For this review, take the finished solid that the model builds, in its own axes (mm). A direction names the side the tool comes from. Give positions to 0.01 mm unless a question says otherwise; leave off trailing zeros. Write each loop counter-clockwise with the first axis right and the second up, starting at its lowest first coordinate (ties: lowest second). Pieces come first, ordered by that corner, then holes. Notation, with made-up numbers: M 47,65 L 66,65 A12 ccw 66,80 Z; hole C 10,71.25 d11. An arc over 180 degrees is marked long. Use one line per item in the form item = value. Start each with the question number.
Q1. Consider section A-A on z = 28. Write out the cut boundary in (x, y).
Q2. Consider section D-D on z = 125. Write out the cut boundary in (x, y).
Q3. Consider section C-C on y = -73. Write out the cut boundary in (x, z).
Q4. For probe 1 along Z at (x, y) = (137.5, -93.5); probe 2 along Y at (x, z) = (129, 45.5), list the stretches that pass through material, from the lowest coordinate up. Write a range as [from, to].
Q5. Tool access review of faces 1 (the flat face through (-101, 1, 50.8)), 2 (the flat face through (-49, -50.8, 101)), 3 (the flat face through (101, -50.8, -1)): name each direction out of +Z, -Z, +X, -X, +Y, -Y from which nothing blocks a thin tool from reaching the whole face with its end or side.
Q6. Consider section B-B on x = 26. Write out the cut boundary in (y, z).
Q7. Clearance check with flat-ended pins moving along their axes: pin 1 Ø1 at (y, z) = (-40.5, -30.5) entering from -X; pin 2 Ø1 at (y, z) = (10.5, 11.5) entering from +X. State where each tip first meets the part, or that it passes through.
```python
from build123d import *

# Parameters (mm, degrees)
F1_W      = 101.6
F1_H      = 101.6
F2_DEPTH  = 50.8
F3_W      = 101.6
F3_H      = 101.6
F4_DEPTH  = 101.6
F5_W      = 101.6
F5_H      = 101.6
F6_DEPTH  = 101.6
F7_W      = 101.6
F7_H      = 101.6
F8_DEPTH  = 101.6
F9_W      = 101.6
F9_H      = 101.6
F10_DEPTH = 101.6


# Not quite as in the source:
# - a variable given as a bare number and used for a length is read in inches; the dataset says mm whatever the document's units were


with BuildPart() as f2:
    # F1 (on Front) → F2 (new body, symmetric)
    with BuildSketch(Plane.XZ):
        Rectangle(F1_W, F1_H)
    extrude(amount=F2_DEPTH, both=True)

    # F3 (on face) → F4 (join)
    with BuildSketch(Plane.XZ.offset(50.8)):
        Rectangle(F3_W, F3_H)
    extrude(amount=F4_DEPTH)

    # F5 (on face) → F6 (join)
    with BuildSketch(Plane.YZ.offset(50.8)):
        with Locations((-101.6, 0)):
            Rectangle(F5_W, F5_H)
    extrude(amount=F6_DEPTH)

    # F7 (on face) → F8 (join)
    with BuildSketch(Plane.XY.offset(50.8)):
        Rectangle(F7_W, F7_H)
    extrude(amount=F8_DEPTH)

    # F9 (on face) → F10 (join)
    with BuildSketch(Plane(origin=(-50.8, 0, 0), x_dir=(0, -1, 0), z_dir=(-1, 0, 0))):
        with Locations((0, 101.6)):
            Rectangle(F9_W, F9_H)
    extrude(amount=F10_DEPTH)


solid = f2.part
```
Working result:
q1.outline = M -50.8,-152.4 L 152.4,-152.4 L 152.4,-50.8 L 50.8,-50.8 L 50.8,50.8 L -50.8,50.8 Z
q2.outline = M -152.4,-50.8 L 50.8,-50.8 L 50.8,50.8 L -152.4,50.8 Z
q3.outline = M -50.8,-50.8 L 152.4,-50.8 L 152.4,50.8 L -50.8,50.8 Z
q4.probe_1 = [-50.8, 50.8]
q4.probe_2 = [-152.4, -50.8]
q5.face_1 = -Z, -X, +Y, -Y
q5.face_2 = +Z, +X, -X, -Y
q5.face_3 = +Z, -Z, +X, +Y
q6.outline = M -152.4,-50.8 L 50.8,-50.8 L 50.8,152.4 L -50.8,152.4 L -50.8,50.8 L -152.4,50.8 Z
q7.pin_1 = -50.8
q7.pin_2 = 50.8
